from build123d import *

# Parameters (mm, degrees)
SKETCH_1_R          = 1.65
EXTRUDE_1_DEPTH     = 3
SKETCH_2_R          = 5.5
SKETCH_2_R_2        = 1.65
EXTRUDE_2_DEPTH     = 1.5
FILLET_2_R          = 50
CUT_EXTRUDE_1_DEPTH = 1.5


with BuildPart() as part:
    # 草图1 → 凸台-拉伸1 (new body)
    with BuildSketch(Plane.XY):
        with BuildLine():
            Line((-2.170396733, 17.309509621), (-2.170396733, -16.690490379))
            ThreePointArc((-2.170396733, -16.690490379), (1.829603267, -25.965407597), (5.829603267, -16.690490379))
            Line((5.829603267, -16.690490379), (5.829603267, 17.309509621))
            ThreePointArc((5.829603267, 17.309509621), (1.829603267, 26.584426838), (-2.170396733, 17.309509621))
        make_face()
        with Locations((1.829603267, 21.084426838)):
            Circle(SKETCH_1_R, mode=Mode.SUBTRACT)
        with Locations((1.829603267, -20.465407597)):
            Circle(SKETCH_1_R, mode=Mode.SUBTRACT)
    extrude(amount=EXTRUDE_1_DEPTH)

    # 草图2 → 凸台-拉伸2 (add)
    # profile 1 of 2: a face of its own
    with BuildSketch(Plane.XY.offset(3)):
        with Locations(Location((1.829603267, 21.084426838, 0), (0, 0, 223.341758227))):
            Circle(SKETCH_2_R)
        Polygon((-1.070396733, 22.758742619), (-1.070396733, 19.410111058), (1.829603267, 17.735795277), (4.729603267, 19.410111058), (4.729603267, 22.758742619), (1.829603267, 24.433058399), align=None, mode=Mode.SUBTRACT)
    # profile 2 of 2: a face of its own
    with BuildSketch(Plane.XY.offset(3)):
        with Locations(Location((1.829603267, -20.465407597, 0), (0, 0, 136.658241773))):
            Circle(SKETCH_2_R)
        with Locations((1.829603267, -20.465407597)):
            Circle(SKETCH_2_R_2, mode=Mode.SUBTRACT)
    extrude(amount=EXTRUDE_2_DEPTH)

    # 圆角2
    # the kernel refuses this fillet: 50 mm, written as the material it adds along each edge
    with BuildSketch(Plane(origin=(-2.170396733, -16.690490379, 0), x_dir=(0, 1, 0), z_dir=(0, 0, 1)), Plane(origin=(5.829603267, 17.309509621, 0), x_dir=(0, -1, 0), z_dir=(0, 0, 1))) as fillet_2_piece_1:
        with BuildLine():
            CenterArc((9.0410884, 50), FILLET_2_R, 256.648815668, 13.351184332)
            ThreePointArc((-2.504862607, 1.351351351), (-1.163505185, 0.840508981), (0, 0))
            Line((0, 0), (9.0410884, 0))
        make_face()
    extrude(amount=3)
    with BuildSketch(Plane(origin=(-2.170396733, 17.309509621, 0), x_dir=(0, -1, 0), z_dir=(0, 0, 1)), Plane(origin=(5.829603267, -16.690490379, 0), x_dir=(0, 1, 0), z_dir=(0, 0, 1))) as fillet_2_piece_2:
        with BuildLine():
            CenterArc((9.0410884, -50), FILLET_2_R, 90, 13.351184332)
            ThreePointArc((-2.504862607, -1.351351351), (-1.163505185, -0.840508981), (0, 0))
            Line((0, 0), (9.0410884, 0))
        make_face()
    extrude(amount=3)

    # 草图5 → 切除-拉伸1 (cut)
    with BuildSketch(Plane(origin=(0, 0, 0), x_dir=(-1, 0, 0), z_dir=(0, 0, -1))):
        Polygon((-4.729603267, -18.791091816), (-4.729603267, -22.139723378), (-1.829603267, -23.814039158), (1.070396733, -22.139723378), (1.070396733, -18.791091816), (-1.829603267, -17.116776036), align=None)
    extrude(amount=-CUT_EXTRUDE_1_DEPTH, mode=Mode.SUBTRACT)


solid = part.part
CAD build for the part. Positions are in the model's coordinates, mm. A direction names the side the tool comes from. Round coordinates to 2 decimals unless told otherwise and drop trailing zeros. Write each loop counter-clockwise with the first axis right and the second up, starting at its lowest first coordinate (ties: lowest second). Pieces come first, ordered by that corner, then holes. Notation, with made-up numbers: M 47,-31.75 L 93,-31.75 A19 ccw 93,-21.75 Z; hole C 38,-35.75 d5. An arc over 180 degrees is marked long. Put each result on its own line as item: value. Start each with the question number.
1) Drill centre lines: probe 1 along Y at (x, z) = (2, 0.7); probe 2 along Y at (x, z) = (3, 3.5); probe 3 along Y at (x, z) = (4.5, 3.35). Where is each one in solid material? Low to high. Write a range as [from, to].
2) Saw through at C-C, the plane x = 4. Write the cut outline in (y, z).
3) Saw through at A-A, the plane z = 3.45. Write the cut outline in (x, y).
4) Pull direction X, two halves, no side cores. Call faces 1 (the flat face through (-2, 21, 4.5)), 2 (the flat face through (-2.17, 0, 1)), 3 (the flat face through (0.359, 18.585, 3.74)): pulls with the +X half, pulls with the -X half, needs draft (parallel to the pull), parting line crosses it, or undercut.
5) 3-axis set-ups, long thin cutter, end or side, ignore diameter. For faces 4 (the flat face through (0.5, 19.6, 3)), 5 (the cylindrical face through (-2.52, -13.54, 1.48)), 6 (the flat face through (2, 0, 0)), 7 (the cylindrical face through (6.16, -13.38, 1.48)), 8 (the flat face through (4.73, -20, 1)): which of +Z, -Z, +X, -X, +Y, -Y reach the whole face in a straight line?
6) Pin check, flat tips, straight feed: pin 1 Ø2 at (y, z) = (-2.5, 1) entering from +X; pin 2 Ø0.9 at (y, z) = (0, 2) entering from -X; pin 3 Ø5.5 at (x, y) = (1.83, -20.47) entering from -Z; pin 4 Ø1.7 at (x, y) = (1.5, -20.5) entering from -Z. Stop position of each tip, or through.
7) Saw through at D-D, the plane y = -5. Write the cut outline in (x, z).
8) Saw through at B-B, the plane z = 0.5. Write the cut outline in (x, y).
Resolved:
1. probe 1: [-25.96, -23.72], [-17.22, 19.44], [22.73, 26.58]
1. probe 2: [-25.84, -21.63], [-19.3, -15.09], [15.71, 18.41], [23.76, 26.46]
1. probe 3: [-25.27, -15.66], [16.28, 19.28], [22.89, 25.89]
2. outline: M -25.52,0 L -22.56,0 L -22.56,1.5 L -18.37,1.5 L -18.37,0 L 26.14,0 L 26.14,4.5 L 23.18,4.5 L 23.18,3 L 18.99,3 L 18.99,4.5 L 16.03,4.5 L 16.03,3 L -15.41,3 L -15.41,4.5 L -25.52,4.5 Z
3. outline: C 1.83,-20.47 d11; C 1.83,21.08 d11; hole M -1.07,19.41 L 1.83,17.74 L 4.73,19.41 L 4.73,22.76 L 1.83,24.43 L -1.07,22.76 Z; hole C 1.83,-20.47 d3.3
4. face 1: needs draft
4. face 2: pulls with the -X half
4. face 3: undercut
5. face 4: +Z
5. face 5: +Z, -Z, -X
5. face 6: -Z, +X, -X, +Y, -Y
5. face 7: +Z, -Z, +X
5. face 8: -Z
6. pin 1: x = 5.83
6. pin 2: x = -2.17
6. pin 3: z = 1.5
6. pin 4: through
7. outline: M -2.17,0 L 5.83,0 L 5.83,3 L -2.17,3 Z
8. outline: M -3.52,-19.2 A5.5 ccw long 7.18,-19.2 A50 cw 5.83,-7.65 L 5.83,8.27 A50 cw 7.18,19.81 A5.5 ccw long -3.52,19.81 A50 cw -2.17,8.27 L -2.17,-7.65 A50 cw Z; hole M -1.07,-22.14 L 1.83,-23.81 L 4.73,-22.14 L 4.73,-18.79 L 1.83,-17.12 L -1.07,-18.79 Z; hole C 1.83,21.08 d3.3
